Design review of the part built by this model. Coordinates are the model's own, in mm. Face numbers are marked on the shaded views. A direction names the side the tool comes from. Coordinates: 2 decimals unless noted, no trailing zeros. Loops run counter-clockwise (first coordinate to the right, second up) from the corner with the lowest first, then second, coordinate; pieces in that order, holes last. Notation, with made-up numbers: (48, -34) -> (81, -34) arc R20 cw to (81, -15) -> close; hole circle Ø1 at (-32.5, 38.25). An arc over 180 degrees is marked (long way). Answer in a Markdown table with one row per item.
```python
from build123d import *

# Parameters (mm, degrees)
SKETCH1_W           = 20
SKETCH1_H           = 105
BOSS_EXTRUDE1_DEPTH = 30
SKETCH2_W           = 40
SKETCH2_H           = 40
BOSS_EXTRUDE2_DEPTH = 20
FILLET1_R           = 10


with BuildPart() as part:
    # Sketch1 → Boss-Extrude1 (new body)
    with BuildSketch(Plane.XY):
        with Locations((-20, -52.5)):
            Rectangle(SKETCH1_W, SKETCH1_H)
    extrude(amount=BOSS_EXTRUDE1_DEPTH)

    # Sketch2 → Boss-Extrude2 (add)
    with BuildSketch(Plane.XY):
        with Locations((-10, -85)):
            Rectangle(SKETCH2_W, SKETCH2_H)
    extrude(amount=-BOSS_EXTRUDE2_DEPTH)

    # Fillet1
    fillet1_edges = [part.edges().sort_by_distance(p)[0] for p in [
        (10, -65, -10),
        (-20, 0, 30),
    ]]
    fillet(fillet1_edges, radius=FILLET1_R)


solid = part.part
```
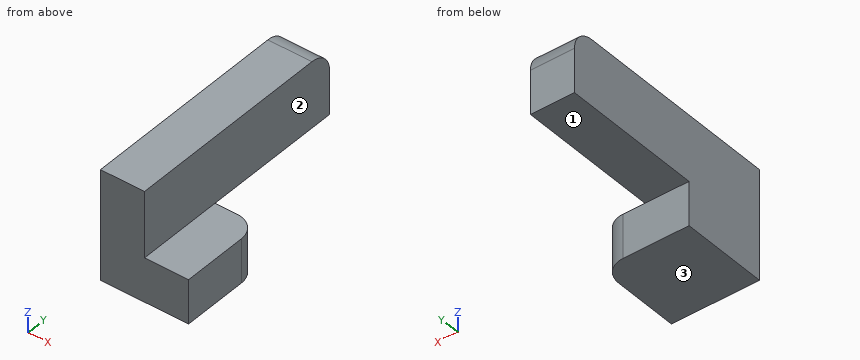
(1) Take a section at C-C on z = 5.5. Give the boundary of the cut face in (x, y), and give its area (3 significant figures).
Evaluation:
| item | result |
|---|---|
| outline | (-30, -105) -> (-10, -105) -> (-10, 0) -> (-30, 0) -> close |
| area | 2,100 mm² |
(2) For pin 1 (6 mm diameter, centred on x = -20, z = -15, fed in from +Y); pin 2 (8 mm diameter, centred on x = -4.5, y = -52.5, fed in from -Z); pin 3 (15 mm diameter, centred on y = -28, z = 9.5, fed in from +X); pin 4 (6 mm diameter, centred on x = -22.5, y = -46.5, fed in from -Z), all flat-tipped, find the tip position at first contact; note any pin that passes through.
Evaluation:
| item | result |
|---|---|
| pin 1 | stops at y = -65 |
| pin 2 | passes through |
| pin 3 | stops at x = -10 |
| pin 4 | stops at z = 0 |
(3) Take a section at B-B on y = -67. Give the boundary of the cut face in (x, z), and give its area (3 significant figures).
Evaluation:
| item | result |
|---|---|
| outline | (-30, -20) -> (6, -20) -> (6, 0) -> (-10, 0) -> (-10, 30) -> (-30, 30) -> close |
| area | 1,320 mm² |
(4) Tool access review of the marked faces 1, 2 and 3: name each direction out of +Z, -Z, +X, -X, +Y, -Y from which nothing blocks a thin tool from reaching the whole face with its end or side.
Evaluation:
| item | result |
|---|---|
| face 1 | -Z, +X, -X, +Y |
| face 2 | +Z, +X, +Y, -Y |
| face 3 | -Z, +X, -X, +Y, -Y |
(5) Take a section at D-D on z = -1. Give the boundary of the cut face in (x, y).
Evaluation:
| item | result |
|---|---|
| outline | (-30, -105) -> (10, -105) -> (10, -75) arc R10 ccw to (0, -65) -> (-30, -65) -> close |
(6) Take a section at A-A on x = -11.5. Give the boundary of the cut face in (y, z), and give its area (3 significant figures).
Evaluation:
| item | result |
|---|---|
| outline | (-105, -20) -> (-65, -20) -> (-65, 0) -> (0, 0) -> (0, 20) arc R10 ccw to (-10, 30) -> (-105, 30) -> close |
| area | 3,930 mm² |
(7) To check wall thickness, follow probe 1 along X at (y, z) = (-79, 7.5); probe 2 along Z at (x, y) = (-9, -69.5); probe 3 along Y at (x, z) = (-25.5, -4). State the ranges of each line that lie inside material, in increasing order.
Evaluation:
| item | result |
|---|---|
| probe 1 | x = -30 to -10 |
| probe 2 | z = -20 to 0 |
| probe 3 | y = -105 to -65 |
